Check sheet for the modelled part. Datum: model origin and axes. Units: mm. A direction names the side the tool comes from. Coordinates: 2 decimals unless noted, no trailing zeros. Write each loop counter-clockwise with the first axis right and the second up, starting at its lowest first coordinate (ties: lowest second). Pieces come first, ordered by that corner, then holes. Notation, with made-up numbers: (87, 74.5) -> (105, 74.5) arc R33 cw to (105, 107.5) -> close; hole circle Ø5 at (37.5, 44.25). An arc over 180 degrees is marked (long way). One line per item, written item: value. Start each with the question number.
1) Gauge pin test, flat ends, axial feed: P1, Ø2.5, axis at x = -2.5, z = 4, coming from the -Y side; P2, Ø1, axis at y = -4.5, z = 9, coming from the +X side; P3, Ø1.1, axis at x = -2.5, y = 10, coming from the -Z side; P4, Ø4.5, axis at x = 0, y = 42, coming from the +Z side. Record the tip position at first contact, or that the pin passes through.
2) Sectioned sample at C-C on x = -42. Enter the section's corners in (y, z).
3) Sectioned sample at A-A on x = 0. Give the number of separate pieces and of enclosed holes in the cut face, plus the area to 3 significant figures.
4) Scan lines: line 1 along X through (y, z) = (0, 0.7); line 2 along Z through (x, y) = (0.5, 12). Record each from-to range of solid material in increasing order. Write a range as [from, to].
5) Draft check along X on faces 1 (the cylindrical face through (47.69, 15.02, 9.54)), 2 (the flat face through (-5.3, 11.5, 0)), 3 (the cylindrical face through (0.74, -3.32, 9.47)). Enter one of: +X half, -X half, draft (parallel to the pull), parting line (faces both ways), or undercut.
6) Set-up check for faces 4 (the flat face through (-10, 0, 2)), 5 (the flat face through (-1, -10, 12)): record each of +Z, -Z, +X, -X, +Y, -Y from which the full face is reachable in a straight line by a thin tool's end or side.
```python
from build123d import *

# Parameters (mm, degrees)
SKETCH1_R              = 14
SKETCH1_R_2            = 12.5
BOSS_EXTRUDE1_DEPTH    = 2
SKETCH2_R              = 14
SKETCH2_W              = 17.67766953
SKETCH2_H              = 17.67766953
BOSS_EXTRUDE2_DEPTH    = 5
SKETCH3_R              = 14
BOSS_EXTRUDE3_DEPTH    = 5
SKETCH6_R              = 50
BOSS_EXTRUDE4_DEPTH    = 5
M8X1_25_TAPPED_HOLE1_D = 6.8
M6X1_0_TAPPED_HOLE1_D  = 5
FILLET1_R              = 6


with BuildPart() as part:
    # Sketch1 → Boss-Extrude1 (new body)
    with BuildSketch(Plane.XY):
        Circle(SKETCH1_R)
        Circle(SKETCH1_R_2, mode=Mode.SUBTRACT)
    extrude(amount=BOSS_EXTRUDE1_DEPTH)

    # Sketch2 → Boss-Extrude2 (add)
    with BuildSketch(Plane.XY.offset(2)):
        Circle(SKETCH2_R)
        Rectangle(SKETCH2_W, SKETCH2_H, mode=Mode.SUBTRACT)
    extrude(amount=BOSS_EXTRUDE2_DEPTH)

    # Sketch3 → Boss-Extrude3 (add)
    with BuildSketch(Plane.XY.offset(7)):
        Circle(SKETCH3_R)
    extrude(amount=BOSS_EXTRUDE3_DEPTH)

    # Sketch6 → Boss-Extrude4 (add)
    with BuildSketch(Plane.XY.offset(12)):
        Circle(SKETCH6_R)
    extrude(amount=-BOSS_EXTRUDE4_DEPTH)

    # M8x1.25 Tapped Hole1 (through all)
    with Locations(Plane.XY.offset(12)):
        with Locations((0, 0)):
            Hole(M8X1_25_TAPPED_HOLE1_D / 2)

    # M6x1.0 Tapped Hole1 (through all)
    with Locations(Plane.XY.offset(12)):
        with Locations((0, 42), (42, 0), (0, -42), (-42, 0)):
            Hole(M6X1_0_TAPPED_HOLE1_D / 2)

    # Fillet1
    fillet1_edges = [part.edges().sort_by_distance(p)[0] for p in [
        (-14, 0, 7),
    ]]
    fillet(fillet1_edges, radius=FILLET1_R)


solid = part.part
```
Answers:
1. P1: stops at y = -15.58
1. P2: stops at x = 49.84
1. P3: stops at z = 2
1. P4: passes through
2. outline: (-27.13, 7) -> (-2.5, 7) -> (-2.5, 12) -> (-27.13, 12) -> close; (2.5, 7) -> (27.13, 7) -> (27.13, 12) -> (2.5, 12) -> close
3. separate pieces: 4
3. enclosed holes: 0
3. area: 489 mm2
4. line 1: x = [-14, -12.5], [12.5, 14]
4. line 2: z = [2, 12]
5. face 1: parting line
5. face 2: draft
5. face 3: undercut
6. face 4: -Z
6. face 5: +Z, +X, -X, +Y, -Y
